Can you work these out from the drawing? Everything is in mm from the part's minimum corner. A direction names the side the tool comes from. Round coordinates to 2 decimals unless told otherwise and drop trailing zeros. Order: outer loops, then holes, each group sorted by start corner. A loop starts at its lowest first (then second) coordinate and runs counter-clockwise, first axis right, second up. Notation, with made-up numbers: (2, -12) -> (20, -12) arc R18 cw to (20, 16) -> close; hole circle Ø5 at (57, 36). An arc over 180 degrees is marked (long way). Use a Markdown table: item, result. Add a question column.
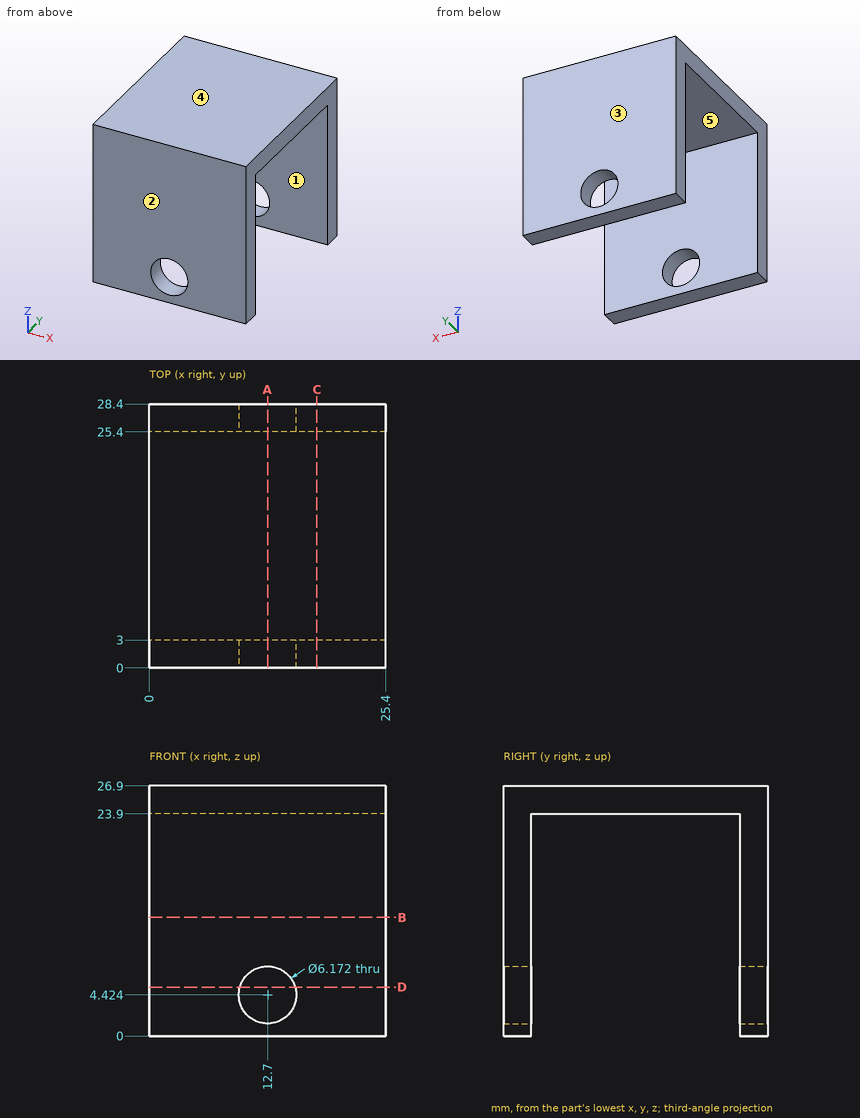
(1) Please list where these lines run through material, in increasing order: probe 1 along Y at (x, z) = (19.5, 19); probe 2 along Z at (x, y) = (12.7, 1.95); probe 3 along Z at (x, y) = (14.75, 23.75). Write a range as from..to.
(2) I want a section at B-B on z = 12.75. List the corners of the cut face in (x, y) for me, and give its area (3 significant figures).
(3) I'm going to push a flat-ended pin straight in: P1, Ø11, axis at x = 11.5, y = 11, coming from the -Z side. Where does the tip first touch, or does it pass through?
(4) If we mould it in two halves opening along Y, with no side actions, what happens to the marked faces 3, 4 and 5? For each: pulls with the +Y half, pulls with the -Y half, needs draft (parallel to the pull), parting line crosses it, or undercut.
(5) I want a section at C-C on x = 18. List the corners of the cut face in (y, z) for me.
(6) I want a section at A-A on x = 12.7. List the corners of the cut face in (y, z) for me.
(7) I want a section at D-D on z = 5.25. List the corners of the cut face in (x, y) for me, and give its area (3 significant figures).
(8) On a 3-axis mill with a long thin cutter (end or side, diameter ignored), from which of +Z, -Z, +X, -X, +Y, -Y can I reach the whole of each face in a straight line? I mean the marked faces 1 and 2. Say none if no direction works.
Output:
| question | item | result |
|---|---|---|
| 1 | probe 1 | 0..3, 25.4..28.4 |
| 1 | probe 2 | 0..1.34, 7.51..26.9 |
| 1 | probe 3 | 23.9..26.9 |
| 2 | outline | (0, 0) -> (25.4, 0) -> (25.4, 3) -> (0, 3) -> close; (0, 25.4) -> (25.4, 25.4) -> (25.4, 28.4) -> (0, 28.4) -> close |
| 2 | area | 152 mm² |
| 3 | P1 | z = 23.9 |
| 4 | face 3 | pulls with the +Y half |
| 4 | face 4 | needs draft |
| 4 | face 5 | undercut |
| 5 | outline | (0, 0) -> (3, 0) -> (3, 23.9) -> (25.4, 23.9) -> (25.4, 0) -> (28.4, 0) -> (28.4, 26.9) -> (0, 26.9) -> close |
| 6 | outline | (0, 0) -> (3, 0) -> (3, 1.34) -> (0, 1.34) -> close; (0, 7.51) -> (3, 7.51) -> (3, 23.9) -> (25.4, 23.9) -> (25.4, 7.51) -> (28.4, 7.51) -> (28.4, 26.9) -> (0, 26.9) -> close; (25.4, 0) -> (28.4, 0) -> (28.4, 1.34) -> (25.4, 1.34) -> close |
| 7 | outline | (0, 0) -> (9.73, 0) -> (9.73, 3) -> (0, 3) -> close; (0, 25.4) -> (9.73, 25.4) -> (9.73, 28.4) -> (0, 28.4) -> close; (15.67, 0) -> (25.4, 0) -> (25.4, 3) -> (15.67, 3) -> close; (15.67, 25.4) -> (25.4, 25.4) -> (25.4, 28.4) -> (15.67, 28.4) -> close |
| 7 | area | 117 mm² |
| 8 | face 1 | -Z, +X, -X |
| 8 | face 2 | +Z, -Z, +X, -X, -Y |
